```python
from build123d import *

# Parameters (mm, degrees)
SKETCH1_R               = 14
BOSS_EXTRUDE1_DEPTH     = 18
SKETCH2_R               = 1.6
CUT_EXTRUDE1_DEPTH      = 18
SKETCH3_R               = 4
CUT_EXTRUDE2_DEPTH      = 10
CUT_EXTRUDE3_DEPTH      = 27.758176321
CUT_EXTRUDE3_DEPTH_BACK = 27.758176321
SKETCH4_R               = 1
CUT_EXTRUDE4_DEPTH      = 27.758176497
CUT_EXTRUDE4_DEPTH_BACK = 27.758176497
SKETCH5_R               = 1


with BuildPart() as part:
    # Sketch1 → Boss-Extrude1 (new body)
    with BuildSketch(Plane(origin=(0, 0, 0), x_dir=(1, 0, 0), z_dir=(0, 1, 0))):
        with Locations(Location((0, 0, 0), (0, 0, 270))):
            Circle(SKETCH1_R)
    extrude(amount=BOSS_EXTRUDE1_DEPTH)

    # Sketch2 → Cut-Extrude1 (cut)
    with BuildSketch(Plane(origin=(0, 18, 0), x_dir=(1, 0, 0), z_dir=(0, 1, 0))):
        with Locations(Location((0, 0, 0), (0, 0, 270))):
            Circle(SKETCH2_R)
    extrude(amount=-CUT_EXTRUDE1_DEPTH, mode=Mode.SUBTRACT)

    # Sketch3 → Cut-Extrude2 (cut)
    with BuildSketch(Plane.XZ):
        with Locations(Location((0, 0, 0), (0, 0, 270))):
            Circle(SKETCH3_R)
    extrude(amount=-CUT_EXTRUDE2_DEPTH, mode=Mode.SUBTRACT)

    # Sketch4 → Cut-Extrude3 (cut, two sides: drawn at the far end of the back side and taken through both)
    with BuildSketch(Plane(origin=(0, 0, 0), x_dir=(0, 0, -1), z_dir=(1, 0, 0)).offset(-CUT_EXTRUDE3_DEPTH_BACK)):
        with Locations((0, 5)):
            Circle(SKETCH4_R)
    extrude(amount=CUT_EXTRUDE3_DEPTH + CUT_EXTRUDE3_DEPTH_BACK, mode=Mode.SUBTRACT)

    # Sketch5 → Cut-Extrude4 (cut, two sides: drawn at the far end of the back side and taken through both)
    with BuildSketch(Plane.XY.offset(-CUT_EXTRUDE4_DEPTH_BACK)):
        with Locations(Location((0, 14, 0), (0, 0, 269.999999966))):
            Circle(SKETCH5_R)
    extrude(amount=CUT_EXTRUDE4_DEPTH + CUT_EXTRUDE4_DEPTH_BACK, mode=Mode.SUBTRACT)


solid = part.part
```
For this review, take the finished solid that the model builds, in its own axes (mm). A direction names the side the tool comes from. Coordinates: 2 decimals unless noted, no trailing zeros. Loops run counter-clockwise (first coordinate to the right, second up) from the corner with the lowest first, then second, coordinate; pieces in that order, holes last.
1. For faces 4 (the cylindrical face through (-1.532, 4.93, -3.695)), 5 (the flat face through (-3, 0, 3)), list the 3-axis set-ups (+Z, -Z, +X, -X, +Y, -Y) from which the entire face can be reached by the end or side of a thin tool; tool diameter is ignored.
2. Mouldability with a two-part tool opening along Z and no side actions: class faces 1 (the cylindrical face through (-13.67, 8.87, -3.03)), 2 (the cylindrical face through (0, 15, 8)), 3 (the flat face through (0, 10, -2)) as +Z half, -Z half, draft (parallel to the pull), parting line (faces both ways), or undercut.
3. For line 1 (Y direction, x = 11.5, z = 0); line 2 (X direction, y = 2, z = -0.25); line 3 (X direction, y = 13.5, z = 0), list the stretches that pass through material, from the lowest coordinate up.
4. Insertion check: P1, Ø3, axis at x = -10.5, y = 3.5, coming from the -Z side; P2, Ø9, axis at x = 1.5, z = -1, coming from the -Y side; P3, Ø3.5, axis at x = 0, z = 0, coming from the -Y side; P4, Ø6, axis at y = 6.5, z = -10, coming from the +X side. Each pin has a flat end and moves straight along its axis. Give the tip position at first contact, or say it passes through.
5. Add section D-D, the plane z = -4.75. Give the boundary of the cut face in (x, y).
6. Add section A-A, the plane x = 0. Give the boundary of the cut face in (y, z), then the cut area to 3 significant figures.
7. Add section B-B, the plane z = 0. Give the boundary of the cut face in (x, y), then the cut area to 3 significant figures.
Result:
1. face 4: -Y
1. face 5: +Z, -Z, +X, -X, -Y
2. face 1: parting line
2. face 2: draft
2. face 3: undercut
3. line 1: y = 0 to 4, 6 to 18
3. line 2: x = -14 to -3.99, 3.99 to 14
3. line 3: x = -14 to -1.6, 1.6 to 14
4. P1: stops at z = -10.72
4. P2: stops at y = 0
4. P3: stops at y = 10
4. P4: stops at x = 12.12
5. outline: (-13.17, 0) - (13.17, 0) - (13.17, 18) - (-13.17, 18) - close; hole circle Ø2 at (0, 14)
6. outline: (0, -14) - (13, -14) - (13, -1.6) - (10, -1.6) - (10, -4) - (0, -4) - close; (0, 4) - (10, 4) - (10, 1.6) - (13, 1.6) - (13, 14) - (0, 14) - close; (15, -14) - (18, -14) - (18, -1.6) - (15, -1.6) - close; (15, 1.6) - (18, 1.6) - (18, 14) - (15, 14) - close
6. area: 349 mm2
7. outline: (-14, 0) - (-4, 0) - (-4, 4) - (-14, 4) - close; (-14, 6) - (-4, 6) - (-4, 10) - (-1.6, 10) - (-1.6, 18) - (-14, 18) - close; (1.6, 10) - (4, 10) - (4, 6) - (14, 6) - (14, 18) - (1.6, 18) - close; (4, 0) - (14, 0) - (14, 4) - (4, 4) - close
7. area: 358 mm2
